Can you work these out from the model? Positions are in its coordinate system, mm. A direction names the side the tool comes from. Give positions to 0.01 mm unless a question says otherwise; leave off trailing zeros. Loops run counter-clockwise (first coordinate to the right, second up) from the corner with the lowest first, then second, coordinate; pieces in that order, holes last. Notation, with made-up numbers: (65.25, 86.5) - (122.25, 86.5) arc R18 cw to (122.25, 112.5) - close; hole circle Ø11 at (33.5, 3). An arc over 180 degrees is marked (long way). Answer in a Markdown table with one row per item.
from build123d import *

# Parameters (mm, degrees)
SKETCH_1_R           = 18.5
SKETCH_1_R_2         = 18
EXTRUDE_1_DEPTH      = 180
CUT_EXTRUDE_1_DEPTH  = 30
SKETCH_5_R           = 1.5
EXTRUDE_2_DEPTH      = 5
SKETCH_8_R           = 1.5
CUT_EXTRUDE_2_DEPTH  = 2
SKETCH_9_R           = 1.5
CUT_EXTRUDE_3_DEPTH  = 2
SKETCH_15_W          = 19.647344242
SKETCH_15_H          = 48.423013506
CUT_EXTRUDE_7_DEPTH  = 208.5
SKETCH_16_W          = 20
SKETCH_16_H          = 0.5
EXTRUDE_4_DEPTH      = 40
SKETCH_17_W          = 20
SKETCH_17_H          = 1
CUT_EXTRUDE_8_DEPTH  = 40
EXTRUDE_8_DEPTH      = 0.5
CUT_EXTRUDE_10_DEPTH = 0.5


with BuildPart() as part:
    # 草图1 → 凸台-拉伸1 (new body)
    with BuildSketch(Plane.XY):
        with Locations(Location((0, 0, 0), (0, 0, 180))):
            Circle(SKETCH_1_R)
        with Locations(Location((0, 0, 0), (0, 0, 180))):
            Circle(SKETCH_1_R_2, mode=Mode.SUBTRACT)
    extrude(amount=EXTRUDE_1_DEPTH)

    # 草图4 → 切除-拉伸1 (cut, symmetric)
    with BuildSketch(Plane(origin=(0, 0, 0), x_dir=(0, 0, -1), z_dir=(1, 0, 0))):
        with BuildLine():
            Line((-2.121320344, -16.378679656), (-8.485281374, -10.014718626))
            ThreePointArc((-8.485281374, -10.014718626), (-4.592201188, -7.41344561), (0, -6.5))
            Line((0, -6.5), (0, -15.5))
            ThreePointArc((0, -15.5), (-1.148050297, -15.728361402), (-2.121320344, -16.378679656))
        make_face()
        with BuildLine():
            Line((-23.744748589, 23.215547635), (0, 23.215547635))
            Line((0, 23.215547635), (0, 20.5))
            ThreePointArc((0, 20.5), (-14.924653862, 17.531301768), (-27.577164466, 9.077164466))
            Line((-27.577164466, 9.077164466), (-33.941125497, 15.441125497))
            ThreePointArc((-33.941125497, 15.441125497), (-29.103701262, 19.670336295), (-23.744748589, 23.215547635))
        make_face()
        with BuildLine():
            Line((-14.849242405, -3.650757595), (-21.213203436, 2.713203436))
            ThreePointArc((-21.213203436, 2.713203436), (-11.480502971, 9.216385975), (0, 11.5))
            Line((0, 11.5), (0, 2.5))
            ThreePointArc((0, 2.5), (-8.03635208, 0.901470183), (-14.849242405, -3.650757595))
        make_face()
    extrude(amount=CUT_EXTRUDE_1_DEPTH, both=True, mode=Mode.SUBTRACT)

    # 草图5 → 凸台-拉伸2 (add, symmetric)
    with BuildSketch(Plane(origin=(0, 0, 0), x_dir=(0, 0, -1), z_dir=(1, 0, 0))):
        with BuildLine():
            Line((-0.190075543, -18), (-2.072124505, -18))
            ThreePointArc((-2.072124505, -18), (1.060660172, -23.060660172), (4.193444848, -18))
            Line((4.193444848, -18), (2.311395887, -18))
            ThreePointArc((2.311395887, -18), (1.060660172, -17.560660172), (-0.190075543, -18))
        make_face()
        with Locations((1.060660172, -19.560660172)):
            Circle(SKETCH_5_R, mode=Mode.SUBTRACT)
    extrude(amount=EXTRUDE_2_DEPTH, both=True)

    # 草图8 → 切除-拉伸2 (cut)
    with BuildSketch(Plane(origin=(3.5, 0, 0), x_dir=(0, 0, -1), z_dir=(1, 0, 0))):
        with BuildLine():
            Line((-0.190075543, -18), (-2.072124505, -18))
            ThreePointArc((-2.072124505, -18), (1.060660172, -23.060660172), (4.193444848, -18))
            Line((4.193444848, -18), (2.311395887, -18))
            ThreePointArc((2.311395887, -18), (1.060660172, -17.560660172), (-0.190075543, -18))
        make_face()
        with Locations((1.060660172, -19.560660172)):
            Circle(SKETCH_8_R, mode=Mode.SUBTRACT)
    extrude(amount=-CUT_EXTRUDE_2_DEPTH, mode=Mode.SUBTRACT)

    # 草图9 → 切除-拉伸3 (cut)
    with BuildSketch(Plane(origin=(-1.5, 0, 0), x_dir=(0, 0, -1), z_dir=(1, 0, 0))):
        with BuildLine():
            Line((-2.072124505, -18), (-0.190075543, -18))
            ThreePointArc((-0.190075543, -18), (1.060660172, -17.560660172), (2.311395887, -18))
            Line((2.311395887, -18), (4.193444848, -18))
            ThreePointArc((4.193444848, -18), (1.060660172, -23.060660172), (-2.072124505, -18))
        make_face()
        with Locations((1.060660172, -19.560660172)):
            Circle(SKETCH_9_R, mode=Mode.SUBTRACT)
    extrude(amount=-CUT_EXTRUDE_3_DEPTH, mode=Mode.SUBTRACT)

    # 草图15 → 切除-拉伸7 (cut, symmetric)
    with BuildSketch(Plane(origin=(0, 0, 0), x_dir=(-1, 0, 0), z_dir=(0, 0, -1))):
        with Locations((9.823672121, -2.226084919)):
            Rectangle(SKETCH_15_W, SKETCH_15_H)
    extrude(amount=CUT_EXTRUDE_7_DEPTH, both=True, mode=Mode.SUBTRACT)

    # 草图16 → 凸台-拉伸4 (add)
    with BuildSketch(Plane(origin=(0, 0, 0), x_dir=(0, 0, -1), z_dir=(1, 0, 0))):
        with Locations((-90, -18.25)):
            Rectangle(SKETCH_16_W, SKETCH_16_H)
        with Locations((-50, -18.25)):
            Rectangle(SKETCH_16_W, SKETCH_16_H)
        with Locations((-130, -18.25)):
            Rectangle(SKETCH_16_W, SKETCH_16_H)
        with Locations((-170, -18.25)):
            Rectangle(SKETCH_16_W, SKETCH_16_H)
    extrude(amount=-EXTRUDE_4_DEPTH)

    # 草图17 → 切除-拉伸8 (cut)
    with BuildSketch(Plane(origin=(0, 0, 0), x_dir=(0, 0, -1), z_dir=(1, 0, 0))):
        with Locations((-110, -18)):
            Rectangle(SKETCH_17_W, SKETCH_17_H)
        with Locations((-150, -18)):
            Rectangle(SKETCH_17_W, SKETCH_17_H)
        with Locations((-70, -18)):
            Rectangle(SKETCH_17_W, SKETCH_17_H)
    extrude(amount=CUT_EXTRUDE_8_DEPTH, mode=Mode.SUBTRACT)

    # 草图20 → 凸台-拉伸8 (add)
    with BuildSketch(Plane.XZ.offset(18.5)):
        with BuildLine():
            Line((0, 59.952777719), (0, 39.932309719))
            ThreePointArc((0, 39.932309719), (-24.004305164, 31.641271223), (-40, 11.916015014))
            Line((-40, 11.916015014), (-40, 44.556181889))
            ThreePointArc((-40, 44.556181889), (-21.280533863, 55.581277174), (0, 59.952777719))
        make_face()
        with BuildLine():
            Line((-40, 68.814162833), (-40, 91.125176599))
            ThreePointArc((-40, 91.125176599), (-20.430552708, 97.494887784), (0, 99.97057031))
            Line((0, 99.97057031), (0, 79.980767144))
            ThreePointArc((0, 79.980767144), (-20.682391226, 76.84186512), (-40, 68.814162833))
        make_face()
        with BuildLine():
            Line((0, 180), (0, 159.99002565))
            ThreePointArc((0, 159.99002565), (-20.167840481, 158.455833888), (-40, 154.483305373))
            Line((-40, 154.483305373), (-40, 175.102068383))
            ThreePointArc((-40, 175.102068383), (-20.132883898, 178.636258798), (0, 180))
        make_face()
        with BuildLine():
            Line((-40, 112.628405695), (-40, 133.686346725))
            ThreePointArc((-40, 133.686346725), (-20.218894936, 138.224000128), (0, 139.978623608))
            Line((0, 139.978623608), (0, 119.975235288))
            ThreePointArc((0, 119.975235288), (-20.297894119, 117.923712576), (-40, 112.628405695))
        make_face()
    extrude(amount=-EXTRUDE_8_DEPTH)

    # 草图21 → 切除-拉伸10 (cut)
    with BuildSketch(Plane.XZ.offset(18.5)):
        with BuildLine():
            Line((0, 79.980767144), (0, 59.952777719))
            ThreePointArc((0, 59.952777719), (-21.280533863, 55.581277174), (-40, 44.556181889))
            Line((-40, 44.556181889), (-40, 68.814162833))
            ThreePointArc((-40, 68.814162833), (-20.682391226, 76.84186512), (0, 79.980767144))
        make_face()
        with BuildLine():
            Line((-40, 91.405123559), (-40, 112.628405695))
            ThreePointArc((-40, 112.628405695), (-20.297894119, 117.923712576), (0, 119.975235288))
            Line((0, 119.975235288), (0, 100.22725283))
            ThreePointArc((0, 100.22725283), (-20.428312001, 97.758177426), (-40, 91.405123559))
        make_face()
        with BuildLine():
            Line((0, 159.99002565), (0, 140.07912782))
            ThreePointArc((0, 140.07912782), (-20.218582252, 138.325773675), (-40, 133.791368433))
            Line((-40, 133.791368433), (-40, 154.483305373))
            ThreePointArc((-40, 154.483305373), (-20.167840481, 158.455833888), (0, 159.99002565))
        make_face()
        with BuildLine():
            Line((-40, 175.084831136), (-40, 180))
            Line((-40, 180), (-40, 184.582306451))
            Line((-40, 184.582306451), (-35.32938599, 184.045292069))
            Line((-35.32938599, 184.045292069), (0, 179.983216215))
            ThreePointArc((0, 179.983216215), (-20.132908432, 178.619348164), (-40, 175.084831136))
        make_face()
    extrude(amount=-CUT_EXTRUDE_10_DEPTH, mode=Mode.SUBTRACT)


solid = part.part
Q1. Imagine slicing it at C-C, the plane z = 24. Write out the boundary of the cut face in (x, y), and give its area (3 significant figures).
Checked values:
| item | result |
|---|---|
| outline | (-40, -18.5) - (-32.46, -18.5) - (-32.46, -18) - (-40, -18) - close; (0, -18.5) arc R18.5 ccw to (13.87, 12.24) - (13.2, 12.24) arc R18 cw to (0, -18) - close |
| area | 24.8 mm² |
Q2. Imagine slicing it at A-A, the plane x = -6.5. Write out the boundary of the cut face in (y, z), and give its area (3 significant figures).
Checked values:
| item | result |
|---|---|
| outline | (-18.5, 39.11) - (-18, 39.11) - (-18, 59.39) - (-18.5, 59.39) - close; (-18.5, 79.55) - (-18, 79.55) - (-18, 99.88) - (-18.5, 99.88) - close; (-18.5, 119.68) - (-18, 119.68) - (-18, 139.82) - (-18.5, 139.82) - close; (-18.5, 159.76) - (-18, 159.76) - (-18, 179.78) - (-18.5, 179.78) - close |
| area | 40.4 mm² |
Q3. Imagine slicing it at B-B, the plane y = 0. Write out the boundary of the cut face in (x, z).
Checked values:
| item | result |
|---|---|
| outline | (18, 0) - (18.5, 0) - (18.5, 9.94) - (18, 9.94) - close; (18, 18.5) - (18.5, 18.5) - (18.5, 180) - (18, 180) - close |
Q4. On a 3-axis mill with a long thin cutter (end or side, diameter ignored), from which of +Z, -Z, +X, -X, +Y, -Y can I reach the whole of each face in a straight line? I mean faces 5 (the face through (8.022, 16.332, 17.543)), 6 (the face through (18.2, -0.5, 18)), 7 (the face through (-19.887, -18.254, 158.494)). Say none if no direction works.
Checked values:
| item | result |
|---|---|
| face 5 | +X, -X, +Y |
| face 6 | +X, -X |
| face 7 | +X, +Y, -Y |
Q5. If I drill on line 1 (Y direction, x = -16, z = 40); line 2 (X direction, y = -11.5, z = 110); line 3 (X direction, y = 6.5, z = 55.5), over which ranges is the centre line in solid material (lowest first)? Write a range as [from, to].
Checked values:
| item | result |
|---|---|
| line 1 | y = [-18.5, -18] |
| line 2 | x = [13.85, 14.49] |
| line 3 | x = [16.79, 17.32] |
Q6. If we mould it in two halves opening along Z, with no side actions, what happens to faces 1 (the face through (-21.401, -18.254, 138.135)), 2 (the face through (-20, -18, 127)), 3 (the face through (-23.708, -18.254, 31.847)), 4 (the face through (-21, -18.25, 55.69))? For each: released by +Z, released by -Z, zero draft, split by the parting line, or undercut.
Checked values:
| item | result |
|---|---|
| face 1 | undercut |
| face 2 | zero draft |
| face 3 | released by -Z |
| face 4 | undercut |
Q7. For pin 1 (8 mm diameter, centred on x = -29.5, z = 74, fed in from -Y); pin 2 (1 mm diameter, centred on y = -10.5, z = 89.5, fed in from +X); pin 3 (8 mm diameter, centred on x = -21.5, z = 63.5, fed in from +Y); pin 4 (0.8 mm diameter, centred on x = 5, z = 1.5, fed in from +Y), each with a flat end and sliding along its axis, tell me the tip position at first contact or that it passes through.
Checked values:
| item | result |
|---|---|
| pin 1 | stops at y = -18.5 |
| pin 2 | stops at x = 15.56 |
| pin 3 | passes through |
| pin 4 | stops at y = 17.92 |
Q8. Imagine slicing it at D-D, the plane x = -19.5. Write out the boundary of the cut face in (y, z).
Checked values:
| item | result |
|---|---|
| outline | (-18.5, 34.43) - (-18, 34.43) - (-18, 56.24) - (-18.5, 56.24) - close; (-18.5, 77.16) - (-18, 77.16) - (-18, 97.96) - (-18.5, 97.96) - close; (-18.5, 118.07) - (-18, 118.07) - (-18, 138.44) - (-18.5, 138.44) - close; (-18.5, 158.55) - (-18, 158.55) - (-18, 178.7) - (-18.5, 178.7) - close |
